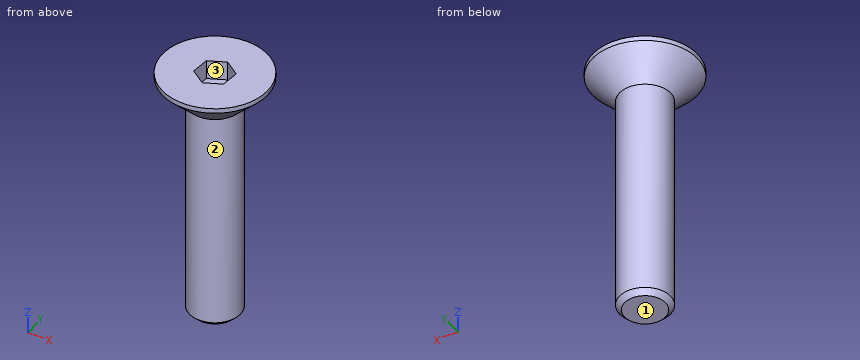
Solid Edge part; units mm, degrees
sketch "Sketch1" plane through (0, 0, 0) normal (0, -1, 0) x (1, 0, 0)
  line L0 (4, 35) -> (4, 0)
  line L1 (4, 0) -> (0, 0)
  line L2 (0, 0) -> (0, 39.96)
  line L3 (0, 39.96) -> (8.215, 39.96)
  line L4 (8.215, 39.96) -> (8.215, 39.215)
  line L5 (4, 35) -> (8.215, 39.215)
revolve "RevolvedProtrusion1" add sketch "Sketch1" angle 360 about axis through (0, 0, 0) along (0, 0, 1)
sketch "Sketch2" plane through (0, 0, 39.96) normal (0, 0, 1) x (0, 1, 0)
  line L0 (1.2028, -2.6242) -> (2.8741, -0.2704)
  line L1 (2.8741, -0.2704) -> (1.6712, 2.3538)
  line L2 (1.6712, 2.3538) -> (-1.2028, 2.6242)
  line L3 (-1.2028, 2.6242) -> (-2.8741, 0.2704)
  line L4 (-2.8741, 0.2704) -> (-1.6712, -2.3538)
  line L5 (-1.6712, -2.3538) -> (1.2028, -2.6242)
extrude "Cutout1" cut sketch "Sketch2" against normal blind 3
cosmetic_thread "Thread1"
chamfer "Chamfer1" distance 0.8 angle 45 1 edges at (-4, 0, 0)
properties material "Stainless steel"
Work out the finished part from the listing and answer in its coordinate system (mm). Face numbers are marked on the shaded views. Coordinates: 2 decimals unless noted, no trailing zeros. Loops run counter-clockwise (first coordinate to the right, second up) from the corner with the lowest first, then second, coordinate; pieces in that order, holes last. Notation, with made-up numbers: (-26, 62) -> (-2, 62) arc R19 ccw to (-2, 76) -> close; hole circle Ø10 at (-32, 14). An arc over 180 degrees is marked (long way). Answer as CSV lines item,"result".
Q1. The part is cut by section A-A on y = 0. Write down the section's boundary in (x, z) (3 decimals).
Findings:
outline,"(-8.215, 39.215) -> (-4, 35) -> (-4, 0.8) -> (-3.2, 0) -> (3.2, 0) -> (4, 0.8) -> (4, 35) -> (8.215, 39.215) -> (8.215, 39.96) -> (2.511, 39.96) -> (2.511, 36.96) -> (-2.511, 36.96) -> (-2.511, 39.96) -> (-8.215, 39.96) -> close"
Q2. Each of these flat-tipped pins is pushed along its axis until it touches: pin 1 (1.6 mm diameter, centred on x = 0.5, y = 1.5, fed in from +Z); pin 2 (3 mm diameter, centred on y = 5, z = 25, fed in from -X); pin 3 (6 mm diameter, centred on x = 1, z = 11, fed in from +Y). Where does it stop, or does it pass through?
Findings:
pin 1,"stops at z = 36.96"
pin 2,"stops at x = -1.94"
pin 3,"stops at y = 4"
Q3. The part is cut by section B-B on z = 14. Write down the section's boundary in (x, y).
Findings:
outline,"circle Ø8 at (0, 0)"
Q4. Find the intervals of material crossed by probe 1 along Y at (x, z) = (0, 28.5); probe 2 along Z at (x, y) = (-1.75, -0.25); probe 3 along Z at (x, y) = (-2, -6.25), in increasing order.
Findings:
probe 1,"y = -4 to 4"
probe 2,"z = 0 to 36.96"
probe 3,"z = 37.56 to 39.96"
Q5. For a pull along X with two mould halves and no side action, classify the marked faces 1, 2 and 3 as +X half, -X half, draft (parallel to the pull), parting line (faces both ways), or undercut.
Findings:
face 1,"draft"
face 2,"parting line"
face 3,"undercut"
